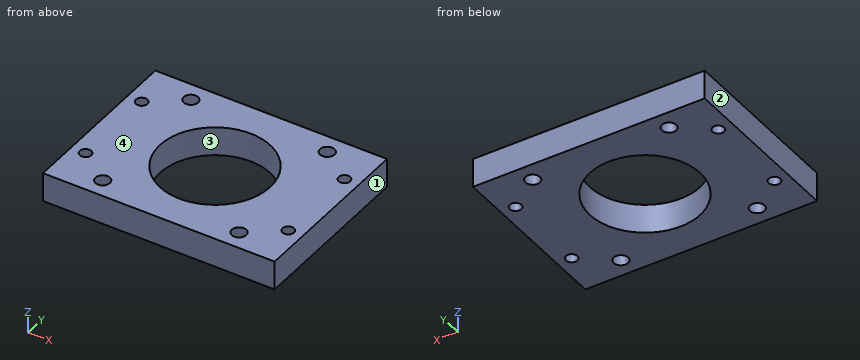
from build123d import *

# Parameters (mm, degrees)
F0_W     = 80
F0_H     = 60
F1_DEPTH = 10
F3_D     = 38.1
F5_D     = 5
F7_D     = 4


with BuildPart() as f1:
    # F0 (on Top) → F1 (new body)
    with BuildSketch(Plane.XY):
        with Locations((40, 30)):
            Rectangle(F0_W, F0_H)
    extrude(amount=F1_DEPTH)

    # F3 (through all)
    with Locations(Plane(origin=(0, 0, 0), x_dir=(1, 0, 0), z_dir=(0, 0, -1))):
        with Locations((40, -30)):
            Hole(F3_D / 2)

    # F5 (through all)
    with Locations(Plane(origin=(0, 0, 0), x_dir=(1, 0, 0), z_dir=(0, 0, -1))):
        with Locations((16.45, -6.45), (63.55, -6.45), (63.55, -53.55), (16.45, -53.55)):
            Hole(F5_D / 2)

    # F7 (through all)
    with Locations(Plane.XY.offset(10)):
        with Locations((5, 45), (75, 45), (75, 15), (5, 15)):
            Hole(F7_D / 2)


solid = f1.part
Geometry: final body of the model. Coordinates: model frame, mm. Face numbers are marked on the shaded views. Round coordinates to 2 decimals unless told otherwise and drop trailing zeros. Order: outer loops, then holes, each group sorted by start corner. A loop starts at its lowest first (then second) coordinate and runs counter-clockwise, first axis right, second up. Notation, with made-up numbers: (5.25, -25) -> (22.25, -25) arc R7 cw to (22.25, -18) -> close; hole circle Ø11 at (9, -40). An arc over 180 degrees is marked (long way). Put each result on its own line as item: value. Start each with the question number.
Q1. Pull-direction query (X, two-part tool) for the marked faces 1, 2, 3 and 4; classes: +X half, -X half, draft (parallel to the pull), parting line (faces both ways), or undercut.
Q2. Section B-B on y = 53.55. Return the cut outline in (x, z).
Q3. Section C-C on x = 56.5. Return the cut outline in (y, z).
Q4. Section D-D on z = 5. Give the number of separate pieces and of enclosed holes in the cut face, and give its area (3 significant figures).
Q5. First-contact query: pin 1 (3.5 mm diameter, centred on x = 75, y = 15, fed in from +Z). Flat tip, straight axial feed; report the tip coordinate or a pass-through.
Q6. Line query: probe 1 along Y at (x, z) = (63.55, 7.75); probe 2 along X at (y, z) = (53.55, 3); probe 3 along X at (y, z) = (7.5, 1.25). Output: solid intervals per line, ascending.
Q7. Section A-A on y = 30. Return the cut outline in (x, z).
Ans:
1. face 1: +X half
1. face 2: -X half
1. face 3: undercut
1. face 4: draft
2. outline: (0, 0) -> (13.95, 0) -> (13.95, 10) -> (0, 10) -> close; (18.95, 0) -> (61.05, 0) -> (61.05, 10) -> (18.95, 10) -> close; (66.05, 0) -> (80, 0) -> (80, 10) -> (66.05, 10) -> close
3. outline: (0, 0) -> (20.48, 0) -> (20.48, 10) -> (0, 10) -> close; (39.52, 0) -> (60, 0) -> (60, 10) -> (39.52, 10) -> close
4. separate pieces: 1
4. enclosed holes: 9
4. area: 3,530 mm2
5. pin 1: passes through
6. probe 1: y = 0 to 3.95, 8.95 to 51.05, 56.05 to 60
6. probe 2: x = 0 to 13.95, 18.95 to 61.05, 66.05 to 80
6. probe 3: x = 0 to 14.18, 18.72 to 61.28, 65.82 to 80
7. outline: (0, 0) -> (20.95, 0) -> (20.95, 10) -> (0, 10) -> close; (59.05, 0) -> (80, 0) -> (80, 10) -> (59.05, 10) -> close
